The drawing under review shows one solid part. Ordinate dimensions are in mm from its lowest x, y, z. Round coordinates to 2 decimals unless told otherwise and drop trailing zeros. Write each loop counter-clockwise with the first axis right and the second up, starting at its lowest first coordinate (ties: lowest second). Pieces come first, ordered by that corner, then holes. Notation, with made-up numbers: (-27.75, -4.75) -> (-12.75, -4.75) arc R13 cw to (-12.75, 11.25) -> close; hole circle Ø1 at (27.25, 45.5). An arc over 180 degrees is marked (long way). Answer in a Markdown table with one row per item. Add a question column.
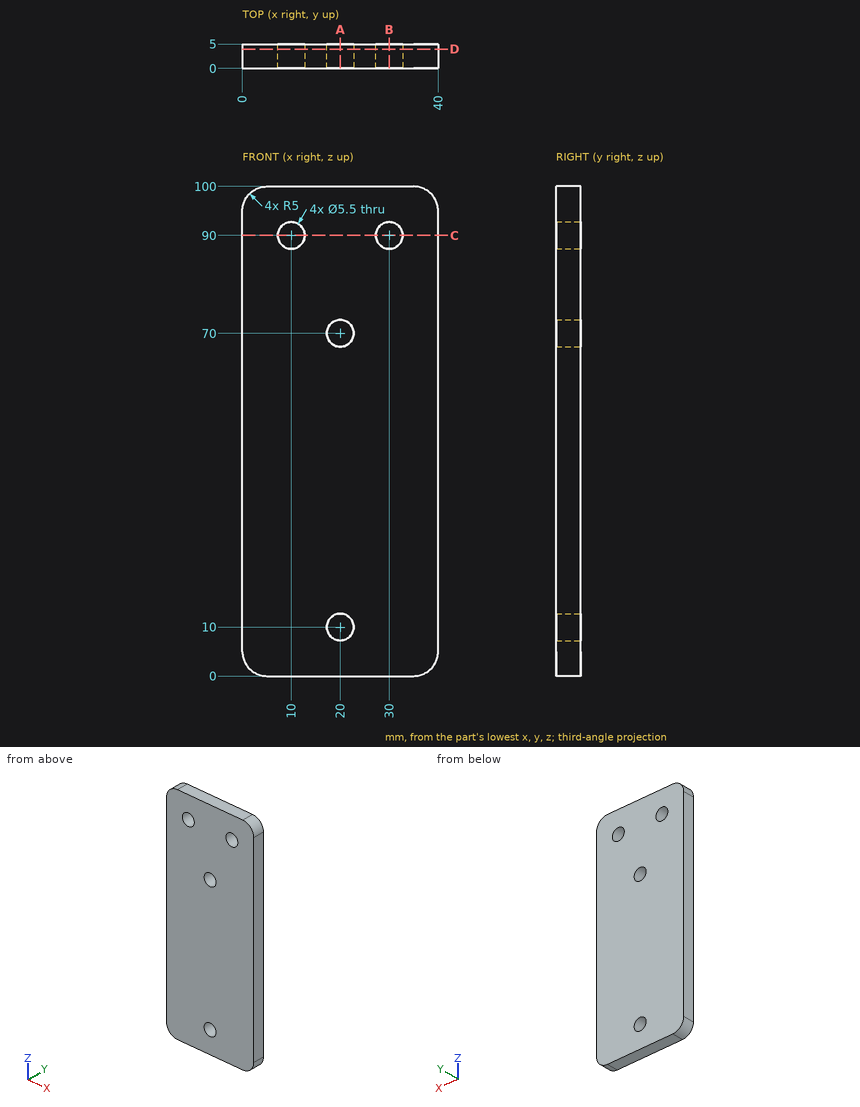
1. Add section B-B on x = 30. Write out the cut boundary in (y, z), plus the area to 4 significant figures.
2. For L1, parallel to Z at x = 20, y = 2.9; L2, parallel to X at y = 3.35, z = 90; L3, parallel to Z at x = 30, y = 2.05, list the stretches that pass through material, from the lowest coordinate up.
3. Add section C-C on z = 90. Write out the cut boundary in (x, y), plus the area to 3 significant figures.
4. Insertion check: pin 1 Ø3.5 at (x, z) = (30, 90) entering from +Y. The pin has a flat end and moves straight along its axis. Give the tip position at first contact, or say it passes through.
5. Add section D-D on y = 3.95. Write out the cut boundary in (x, z), plus the area to 3 significant figures.
6. Add section A-A on x = 20. Write out the cut boundary in (y, z), plus the area to 3 significant figures.
Filled in:
| question | item | result |
|---|---|---|
| 1 | outline | (0, 0) -> (5, 0) -> (5, 87.25) -> (0, 87.25) -> close; (0, 92.75) -> (5, 92.75) -> (5, 100) -> (0, 100) -> close |
| 1 | area | 472.5 mm² |
| 2 | L1 | 0 to 7.25, 12.75 to 67.25, 72.75 to 100 |
| 2 | L2 | 0 to 7.25, 12.75 to 27.25, 32.75 to 40 |
| 2 | L3 | 0 to 87.25, 92.75 to 100 |
| 3 | outline | (0, 0) -> (7.25, 0) -> (7.25, 5) -> (0, 5) -> close; (12.75, 0) -> (27.25, 0) -> (27.25, 5) -> (12.75, 5) -> close; (32.75, 0) -> (40, 0) -> (40, 5) -> (32.75, 5) -> close |
| 3 | area | 145 mm² |
| 4 | pin 1 | through |
| 5 | outline | (0, 5) arc R5 ccw to (5, 0) -> (35, 0) arc R5 ccw to (40, 5) -> (40, 95) arc R5 ccw to (35, 100) -> (5, 100) arc R5 ccw to (0, 95) -> close; hole circle Ø5.5 at (10, 90); hole circle Ø5.5 at (20, 10); hole circle Ø5.5 at (20, 70); hole circle Ø5.5 at (30, 90) |
| 5 | area | 3,880 mm² |
| 6 | outline | (0, 0) -> (5, 0) -> (5, 7.25) -> (0, 7.25) -> close; (0, 12.75) -> (5, 12.75) -> (5, 67.25) -> (0, 67.25) -> close; (0, 72.75) -> (5, 72.75) -> (5, 100) -> (0, 100) -> close |
| 6 | area | 445 mm² |
